Check sheet for the drawn part. Datum: minimum x, y, z corner. Units: mm. A direction names the side the tool comes from. Give positions to 0.01 mm unless a question says otherwise; leave off trailing zeros. Order: outer loops, then holes, each group sorted by start corner. A loop starts at its lowest first (then second) coordinate and runs counter-clockwise, first axis right, second up. Notation, with made-up numbers: M -18,-12 L 16,-12 A23 cw 16,19 Z; hole C 9.5,63.5 d8. An arc over 180 degrees is marked long. Put each result on its own line as item: value. Start each with the question number.
Q1. Go/stop test with flat-tipped pins: pin 1 (1 mm diameter, centred on x = 12.5, y = 15.5, fed in from -Z); pin 2 (3 mm diameter, centred on x = 6, y = 6.5, fed in from +Z); pin 3 (10 mm diameter, centred on y = 13.5, z = 5, fed in from +X). Record where each tip stops, or that it passes through.
Q2. Section check A-A on z = 15. Record the cut outline in (x, y).
Q3. Access from +Z, -Z, +X, -X, +Y, -Y to the whole of each face (thin tool, end or side, straight path). Record for the marked faces 1 and 2.
Q4. Material ranges on L1, parallel to Y at x = 1.3, z = 15; L2, parallel to Z at x = 11.25, y = 15; L3, parallel to Z at x = 18.5, y = 15, recorded low to high.
Q5. Section check B-B on x = 2. Record the cut outline in (y, z).
Q6. Section check D-D on z = 5. Record the cut outline in (x, y), then the cut area to 3 significant figures.
Q7. Section check C-C on y = 14.5. Record the cut outline in (x, z).
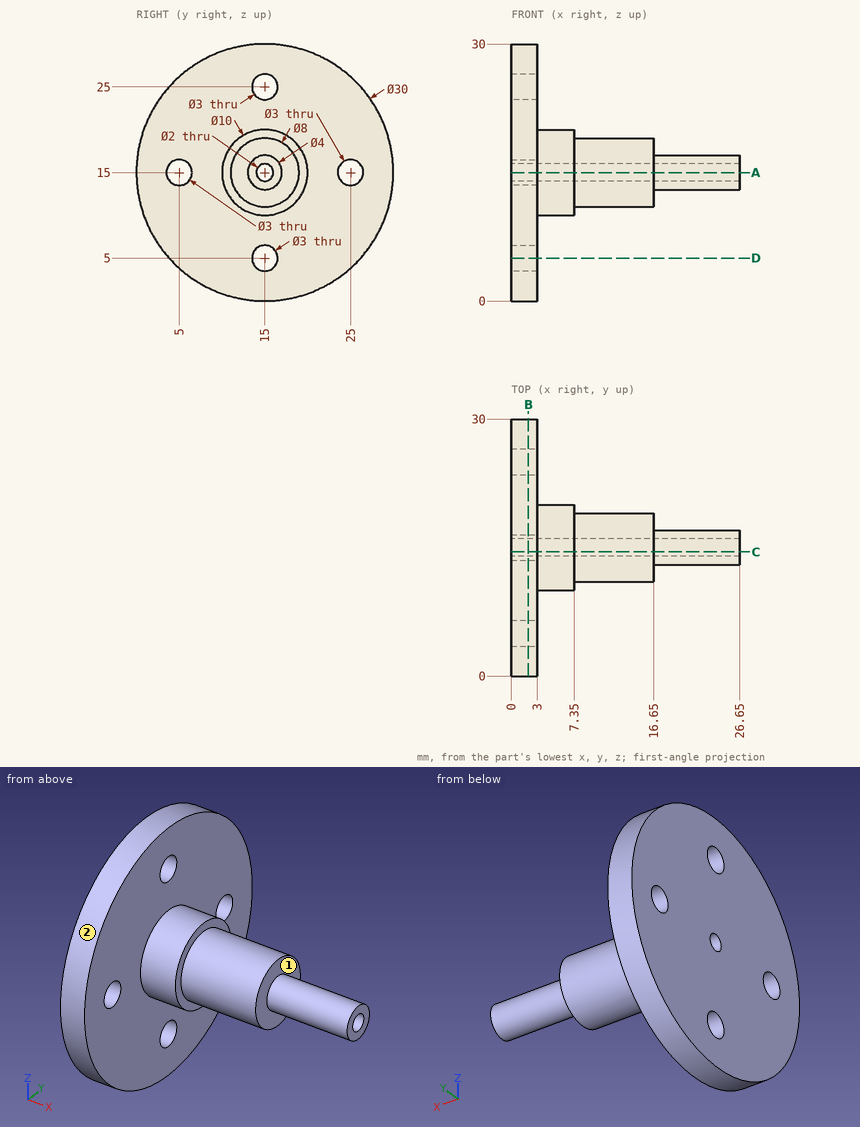
Results found:
1. pin 1: stops at z = 11
1. pin 2: passes through
1. pin 3: stops at x = 3
2. outline: M 0,0 L 3,0 L 3,3.5 L 0,3.5 Z; M 0,6.5 L 3,6.5 L 3,10 L 7.35,10 L 7.35,11 L 16.65,11 L 16.65,13 L 26.65,13 L 26.65,14 L 0,14 Z; M 0,16 L 26.65,16 L 26.65,17 L 16.65,17 L 16.65,19 L 7.35,19 L 7.35,20 L 3,20 L 3,23.5 L 0,23.5 Z; M 0,26.5 L 3,26.5 L 3,30 L 0,30 Z
3. face 1: +X
3. face 2: +X, -X
4. L1: y = 0 to 3.5, 6.5 to 14, 16 to 23.5, 26.5 to 30
4. L2: z = 11 to 14, 16 to 19
4. L3: z = 13 to 14, 16 to 17
5. outline: C 15,15 d30; hole C 5,15 d3; hole C 15,5 d3; hole C 15,25 d3; hole C 15,15 d2; hole C 25,15 d3
6. outline: M 0,3.82 L 3,3.82 L 3,13.5 L 0,13.5 Z; M 0,16.5 L 3,16.5 L 3,26.18 L 0,26.18 Z
6. area: 58.1 mm^2
7. outline: M 0,0.01 L 3,0.01 L 3,3.59 L 0,3.59 Z; M 0,6.41 L 3,6.41 L 3,10.03 L 7.35,10.03 L 7.35,11.03 L 16.65,11.03 L 16.65,13.06 L 26.65,13.06 L 26.65,14.13 L 0,14.13 Z; M 0,15.87 L 26.65,15.87 L 26.65,16.94 L 16.65,16.94 L 16.65,18.97 L 7.35,18.97 L 7.35,19.97 L 3,19.97 L 3,23.59 L 0,23.59 Z; M 0,26.41 L 3,26.41 L 3,29.99 L 0,29.99 Z
